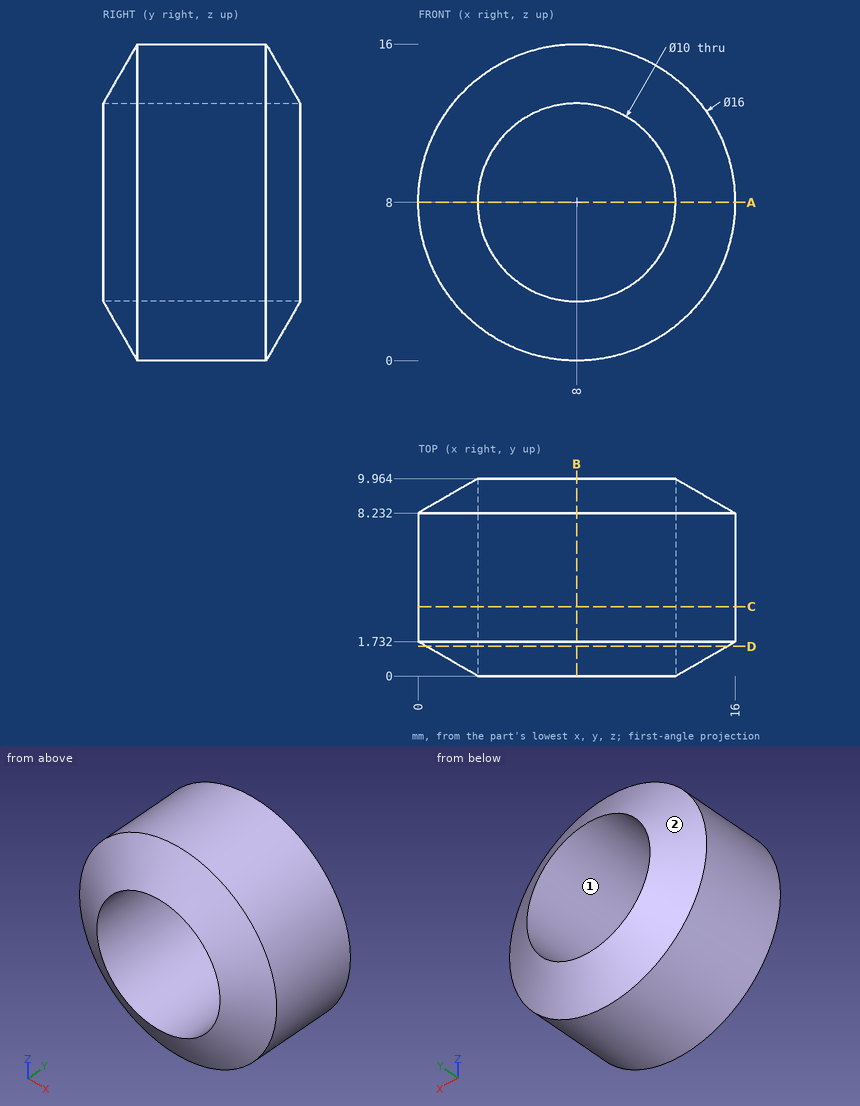
Could you check a few things on this drawing? It's one solid part, dimensions in mm from its lowest x, y, z. Coordinates: 2 decimals unless noted, no trailing zeros. Order: outer loops, then holes, each group sorted by start corner. A loop starts at its lowest first (then second) coordinate and runs counter-clockwise, first axis right, second up. Notation, with made-up numbers: M -28.5,38.5 L 2.5,38.5 A29 cw 2.5,67.5 Z; hole C 77,63.5 d10. An arc over 180 degrees is marked long. Answer as a JSON object with one key per item and string values. Group by question number.
(1) Suppose I cut it at B-B, the plane x = 8. Please give me the cut outline in (y, z).
(2) Suppose I cut it at D-D, the plane y = 1.5. Please give me the cut outline in (x, z).
(3) If we mould it in two halves opening along Z, with no side actions, what happens to the marked faces 1 and 2? For each: released by +Z, released by -Z, zero draft, split by the parting line, or undercut.
(4) I need wall thicknesses on probe 1 along X at (y, z) = (2.5, 8); probe 2 along Z at (x, y) = (11.5, 2.5); probe 3 along Z at (x, y) = (6.25, 9). Which ranges of each line are inside material? Lowest first, please.
(5) For pin 1 (1.5 mm diameter, centred on x = 11.5, y = 7, fed in from -Z), with a flat end and sliding along its axis, tell me the tip position at first contact or that it passes through.
(6) Suppose I cut it at C-C, the plane y = 3.5. Please give me the cut outline in (x, z).
(7) Suppose I cut it at A-A, the plane z = 8. Please give me the cut outline in (x, y), then the cut area to 3 significant figures.
Values found:
{
 "1": {"outline": "M 0,3 L 1.73,0 L 8.23,0 L 9.96,3 Z; M 0,13 L 9.96,13 L 8.23,16 L 1.73,16 Z"},
 "2": {"outline": "C 8,8 d15.2; hole C 8,8 d10"},
 "3": {"face 1": "undercut", "face 2": "split by the parting line"},
 "4": {"probe 1": "x = 0 to 3, 13 to 16", "probe 2": "z = 0.81 to 4.43, 11.57 to 15.19", "probe 3": "z = 1.56 to 3.32, 12.68 to 14.44"},
 "5": {"pin 1": "stops at z = 0.49"},
 "6": {"outline": "C 8,8 d16; hole C 8,8 d10"},
 "7": {"outline": "M 0,1.73 L 3,0 L 3,9.96 L 0,8.23 Z; M 13,0 L 16,1.73 L 16,8.23 L 13,9.96 Z", "area": "49.4 mm^2"}
}
